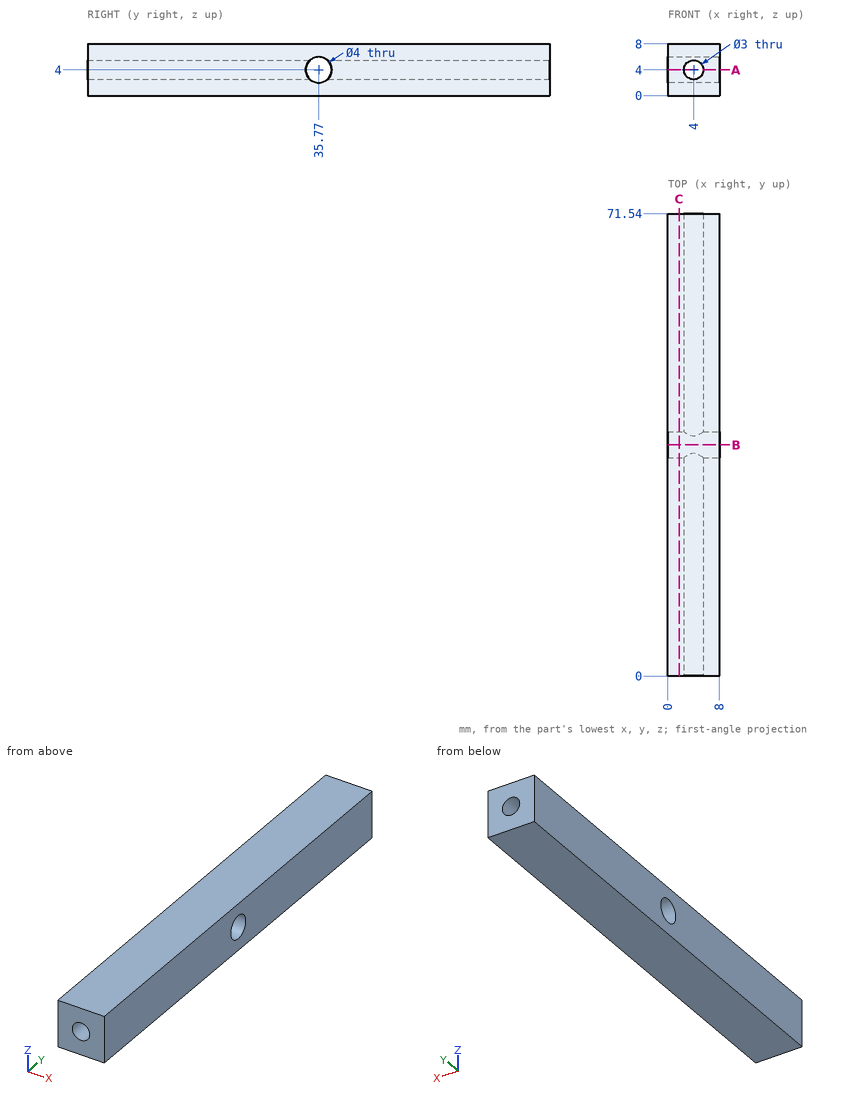
The drawing under review shows one solid part. Ordinate dimensions are in mm from its lowest x, y, z. Round coordinates to 2 decimals unless told otherwise and drop trailing zeros. Order: outer loops, then holes, each group sorted by start corner. A loop starts at its lowest first (then second) coordinate and runs counter-clockwise, first axis right, second up. Notation, with made-up numbers: M 86,12.5 L 145,12.5 A13 ccw 145,33.5 Z; hole C -29.5,87 d6. An arc over 180 degrees is marked long. Answer as CSV lines item,"result". Start each with the question number.
1) For pin 1 Ø2.5 at (x, z) = (4, 4) entering from +Y, flat-tipped, find the tip position at first contact; note if it passes through.
2) Add section A-A (z = 4). Give the boundary of the cut face in (x, y).
3) Add section C-C (x = 1.75). Give the boundary of the cut face in (y, z).
4) Add section B-B (y = 35.77). Give the boundary of the cut face in (x, z).
5) Wall thickness on line 1 along X through (y, z) = (58.5, 4); line 2 along Z through (x, y) = (5, 56); line 3 along Y through (x, z) = (2.5, 2.25): over which ranges is each line inside the solid? List them lowest first. Write a range as [from, to].
Resolved:
1,pin 1,"through"
2,outline,"M 0,0 L 2.5,0 L 2.5,33.77 L 0,33.77 Z; M 0,37.77 L 2.5,37.77 L 2.5,71.54 L 0,71.54 Z; M 5.5,0 L 8,0 L 8,33.77 L 5.5,33.77 Z; M 5.5,37.77 L 8,37.77 L 8,71.54 L 5.5,71.54 Z"
3,outline,"M 0,0 L 71.54,0 L 71.54,8 L 0,8 Z; hole C 35.77,4 d4"
4,outline,"M 0,0 L 8,0 L 8,2 L 0,2 Z; M 0,6 L 8,6 L 8,8 L 0,8 Z"
5,line 1,"[0, 2.5], [5.5, 8]"
5,line 2,"[0, 2.88], [5.12, 8]"
5,line 3,"[0, 34.8], [36.74, 71.54]"
